The figure shows three views and two pictorial views of one solid part (mm, origin at its lowest corner). Answer the questions. Give positions to 0.01 mm unless a question says otherwise; leave off trailing zeros. Loops run counter-clockwise (first coordinate to the right, second up) from the corner with the lowest first, then second, coordinate; pieces in that order, holes last. Notation, with made-up numbers: M 47,-27.75 L 81,-27.75 A17 ccw 81,-20.75 Z; hole C 29,-1 d11. An arc over 180 degrees is marked long. One line per item, written item: value. Start each with the question number.
Q1. Flat-ended cylindrical pins translate along their axes: pin 1 (2.5 mm diameter, centred on x = 5, y = 48.5, fed in from -Z); pin 2 (1.5 mm diameter, centred on y = 2.5, z = 3, fed in from +X); pin 3 (1.5 mm diameter, centred on x = 50, z = 4, fed in from -Y); pin 4 (2.5 mm diameter, centred on x = 62, z = 2.5, fed in from +Y). Find the tip coordinate at first contact, or state that the pin passes through.
Q2. A cutting plane is placed at A-A, the plane y = 48.5. Determine the outline of the cut face in (x, z).
Q3. Consider L1, parallel to X at y = 48.5, z = 2; L2, parallel to Y at x = 5, z = 1.5; L3, parallel to Y at x = 74.5, z = 2.55. Determine where each line is inside the solid, lowest interval first.
Q4. A cutting plane is placed at B-B, the plane z = 4.1. Determine the outline of the cut face in (x, y).
Q5. A cutting plane is placed at C-C, the plane x = 73.5. Determine the outline of the cut face in (y, z).
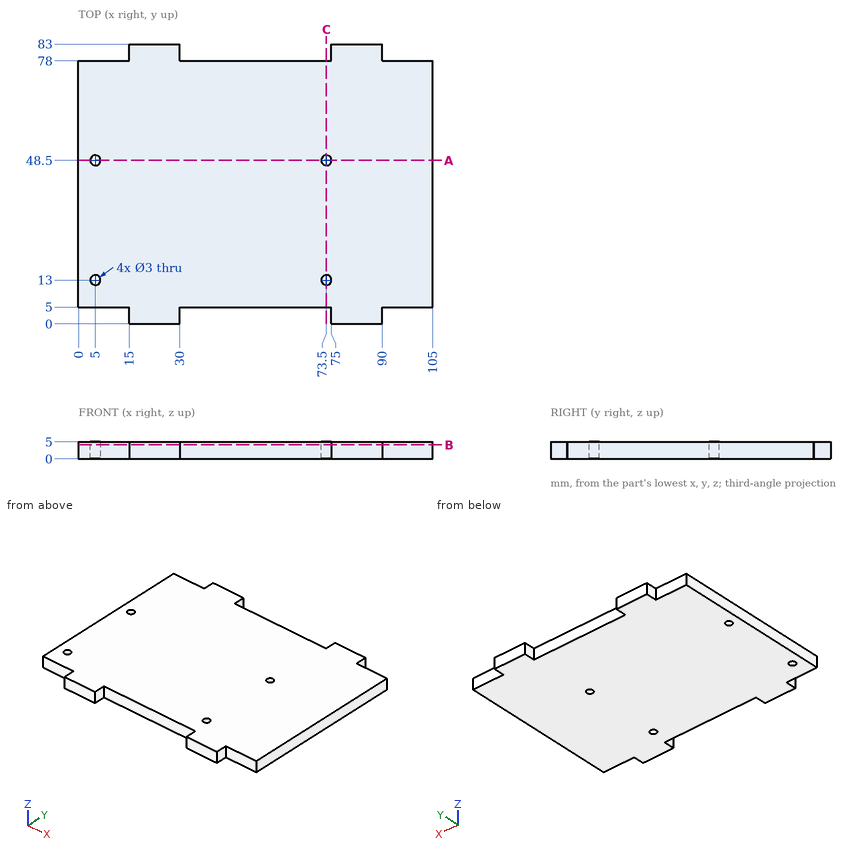
Answer block:
1. pin 1: through
1. pin 2: x = 90
1. pin 3: y = 5
1. pin 4: y = 78
2. outline: M 0,0 L 3.5,0 L 3.5,5 L 0,5 Z; M 6.5,0 L 72,0 L 72,5 L 6.5,5 Z; M 75,0 L 105,0 L 105,5 L 75,5 Z
3. L1: 0 to 3.5, 6.5 to 72, 75 to 105
3. L2: 5 to 11.5, 14.5 to 47, 50 to 78
3. L3: 5 to 11.88, 14.12 to 47.38, 49.62 to 78
4. outline: M 0,5 L 15,5 L 15,0 L 30,0 L 30,5 L 75,5 L 75,0 L 90,0 L 90,5 L 105,5 L 105,78 L 90,78 L 90,83 L 75,83 L 75,78 L 30,78 L 30,83 L 15,83 L 15,78 L 0,78 Z; hole C 5,13 d3; hole C 5,48.5 d3; hole C 73.5,13 d3; hole C 73.5,48.5 d3
5. outline: M 5,0 L 11.5,0 L 11.5,5 L 5,5 Z; M 14.5,0 L 47,0 L 47,5 L 14.5,5 Z; M 50,0 L 78,0 L 78,5 L 50,5 Z
